```python
from build123d import *

# Parameters (mm, degrees)
SKETCH_1_W          = 100
SKETCH_1_H          = 40
EXTRUDE_1_DEPTH     = 80
SKETCH_3_W          = 30
SKETCH_3_H          = 30
CUT_EXTRUDE_2_DEPTH = 20
SKETCH_6_R          = 5
EXTRUDE_2_DEPTH     = 20
SKETCH_7_W          = 70
SKETCH_7_H          = 80
CUT_EXTRUDE_3_DEPTH = 40
FILLET_1_R          = 30
FILLET_2_R          = 30
FILLET_3_R          = 30
FILLET_4_R          = 20
FILLET_5_R          = 20


with BuildPart() as part:
    # 草圖1 → 填料-伸長1 (new body)
    with BuildSketch(Plane(origin=(0, 0, 0), x_dir=(1, 0, 0), z_dir=(0, 1, 0))):
        Rectangle(SKETCH_1_W, SKETCH_1_H)
    extrude_1 = extrude(amount=EXTRUDE_1_DEPTH)

    # 草圖3 → 除料-伸長2 (cut)
    with BuildSketch(Plane.XY.offset(20)):
        with Locations((-35, 15)):
            Rectangle(SKETCH_3_W, SKETCH_3_H)
        with Locations((35, 15)):
            Rectangle(SKETCH_3_W, SKETCH_3_H)
    cut_extrude_2 = extrude(amount=-CUT_EXTRUDE_2_DEPTH, mode=Mode.SUBTRACT)

    # 草圖6 → 填料-伸長2 (add)
    with BuildSketch(Plane.XY):
        with Locations((-43, 7)):
            Circle(SKETCH_6_R)
        with Locations((43, 7)):
            Circle(SKETCH_6_R)
    extrude_2 = extrude(amount=EXTRUDE_2_DEPTH)

    # 鏡射3: 填料-伸長1, 除料-伸長2, 填料-伸長2 across plane
    add(extrude_1.mirror(Plane(origin=(-50, 80, 20), x_dir=(1, 0, 0), z_dir=(0, 0, -1))))
    add(cut_extrude_2.mirror(Plane(origin=(-50, 80, 20), x_dir=(1, 0, 0), z_dir=(0, 0, -1))), mode=Mode.SUBTRACT)
    add(extrude_2.mirror(Plane(origin=(-50, 80, 20), x_dir=(1, 0, 0), z_dir=(0, 0, -1))))

    # 草圖7 → 除料-伸長3 (cut)
    with BuildSketch(Plane(origin=(0, 80, 0), x_dir=(1, 0, 0), z_dir=(0, 1, 0))):
        with Locations((-15, -20)):
            Rectangle(SKETCH_7_W, SKETCH_7_H)
    extrude(amount=-CUT_EXTRUDE_3_DEPTH, mode=Mode.SUBTRACT)

    # 圓角1
    fillet_1_edges = [part.edges().sort_by_distance(p)[0] for p in [
        (50, 80, 20),
    ]]
    fillet(fillet_1_edges, radius=FILLET_1_R - 0.0001)  # a hair under: the kernel refuses the full size

    # 圓角2
    fillet_2_edges = [part.edges().sort_by_distance(p)[0] for p in [
        (50, 25.00005, 60),
        (41.213232725, 71.213232725, 60),
    ]]
    fillet(fillet_2_edges, radius=FILLET_2_R - 0.0001)  # a hair under: the kernel refuses the full size

    # 圓角3
    fillet_3_edges = [part.edges().sort_by_distance(p)[0] for p in [
        (50, 25.00005, -20),
        (41.213232725, 71.213232725, -20),
    ]]
    fillet(fillet_3_edges, radius=FILLET_3_R - 0.0001)  # a hair under: the kernel refuses the full size

    # 圓角4
    fillet_4_edges = [part.edges().sort_by_distance(p)[0] for p in [
        (-15, 40, 60),
    ]]
    fillet(fillet_4_edges, radius=FILLET_4_R)

    # 圓角5
    fillet_5_edges = [part.edges().sort_by_distance(p)[0] for p in [
        (-15, 40, -20),
    ]]
    fillet(fillet_5_edges, radius=FILLET_5_R)


solid = part.part
```
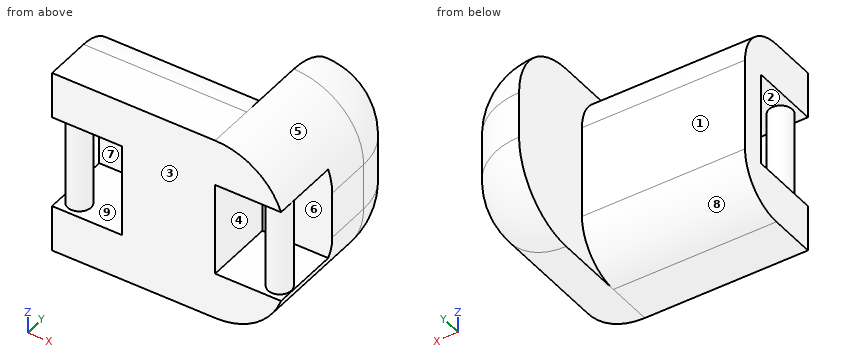
For this review, take the finished solid that the model builds, in its own axes (mm). Face numbers are marked on the shaded views. A direction names the side the tool comes from. Round coordinates to 2 decimals unless told otherwise and drop trailing zeros. Write each loop counter-clockwise with the first axis right and the second up, starting at its lowest first coordinate (ties: lowest second). Pieces come first, ordered by that corner, then holes. Notation, with made-up numbers: (71.5, 73.25) - (111.5, 73.25) arc R30 ccw to (111.5, 112.25) - close; hole circle Ø11 at (69.5, 5.5). An arc over 180 degrees is marked (long way). Put each result on its own line as item: value.
Q1. Mouldability with a two-part tool opening along Y and no side actions: class the marked faces 1, 2, 3 and 4 as released by +Y, released by -Y, zero draft, split by the parting line, or undercut.
Solved:
face 1: released by +Y
face 2: undercut
face 3: released by -Y
face 4: zero draft
Q2. Wall thickness on probe 1 along Z at (x, y) = (-37.5, 19.5); probe 2 along X at (y, z) = (3.5, 10.5); probe 3 along X at (y, z) = (14, 8.5): over which ranges is each line inside the solid? List them lowest first.
Solved:
probe 1: z = -20 to 0, 40 to 60
probe 2: x = -46.57 to -39.43, -20 to 20, 39.43 to 46.57
probe 3: x = -20 to 20
Q3. We need section B-B (y = 7). Give the boundary of the cut face in (x, z).
Solved:
outline: (-50, -20) - (20, -20) arc R30 ccw to (48.28, 0) - (48, 0) - (48, 40) - (48.28, 40) arc R30 ccw to (20, 60) - (-50, 60) - (-50, 40) - (-48, 40) - (-48, 0) - (-50, 0) - close; hole (-38, 0) - (-20, 0) - (-20, 40) - (-38, 40) - close; hole (20, 0) - (38, 0) - (38, 40) - (20, 40) - close
Q4. We need section C-C (x = -23). Give the boundary of the cut face in (y, z).
Solved:
outline: (0, -20) - (20, -20) arc R20 ccw to (40, 0) - (40, 40) arc R20 ccw to (20, 60) - (0, 60) - (0, 40) - (30, 40) - (30, 0) - (0, 0) - close
Q5. We need section A-A (x = -43). Give the boundary of the cut face in (y, z), and give its area (3 significant figures).
Solved:
outline: (0, -20) - (20, -20) arc R20 ccw to (40, 0) - (40, 40) arc R20 ccw to (20, 60) - (0, 60) - (0, 40) - (2, 40) - (2, 0) - (0, 0) - close; hole (12, 0) - (30, 0) - (30, 40) - (12, 40) - close
area: 2,230 mm2
Q6. Insertion check: pin 1 Ø12 at (x, z) = (-15.5, 26) entering from +Y; pin 2 Ø8 at (x, y) = (-35, 25) entering from +Z (3 decimals); pin 3 Ø8.5 at (x, y) = (34.5, 21.5) entering from +Z. Each pin has a flat end and moves straight along its axis. Give the tip position at first contact, or say it passes through.
Solved:
pin 1: stops at y = 40
pin 2: stops at z = 59.975
pin 3: stops at z = 58.19
Q7. We need section D-D (z = 37.5). Count the separate pieces of the cut face and the enclosed holes in it, and give its area (3 significant figures).
Solved:
separate pieces: 3
enclosed holes: 0
area: 3,300 mm2
Q8. Machinability: for the marked faces 5, 6, 7, 8 and 9, which of the approach directions +Z, -Z, +X, -X, +Y, -Y give a long, thin tool a straight path to every point of the face, cutting with its end or side? Answer none if there is none.
Solved:
face 5: +Z, +X, +Y, -Y
face 6: +X
face 7: -X
face 8: -Z, -X, +Y
face 9: none
